Could you check a few things on this model? Use its own coordinates, in mm. A direction names the side the tool comes from. Coordinates: 2 decimals unless noted, no trailing zeros. Write each loop counter-clockwise with the first axis right and the second up, starting at its lowest first coordinate (ties: lowest second). Pieces come first, ordered by that corner, then holes.
Autodesk Inventor part; units mm, degrees
ref_plane "YZ Plane" through (0, 0, 0) normal (1, 0, 0) x (0, 1, 0)
ref_plane "XZ Plane" through (0, 0, 0) normal (0, 1, 0) x (-1, 0, 0)
ref_plane "XY Plane" through (0, 0, 0) normal (0, 0, 1) x (1, 0, 0)
sketch "Boceto1" plane through (0, 0, 0) normal (0, 0, 1) x (1, 0, 0)
  line L0 (-80, -30) -> (80, -30)
  line L1 (80, 30) -> (-80, 30)
  line L2 (-80, -30) -> (80, 30) construction
  line L3 (80, -30) -> (-80, 30) construction
  line L4 (0, -42) -> (0, 42) construction
  line L5 (-112, 0) -> (112, 0) construction
  arc A0 (-60, -10) -> (-60, 10) centre (-60, 0) ccw
  line L6 (-80, 10) -> (-60, 10)
  line L7 (-80, -10) -> (-60, -10)
  arc A1 (60, 10) -> (60, -10) centre (60, 0) ccw
  line L8 (80, 10) -> (60, 10)
  line L9 (80, -10) -> (60, -10)
  line L10 (-80, 30) -> (-80, 10)
  line L11 (-80, -10) -> (-80, -30)
  line L12 (80, -30) -> (80, -10)
  line L13 (80, 10) -> (80, 30)
  point P0 (0, 0)
  dimension "d2" = 160
  dimension "d3" = 60
  dimension "d4" = 20
  dimension "d6" = 20
  dimension "d7" = 20
extrude "Extrusión1" add sketch "Boceto1" along normal blind 20
sketch "Boceto2" plane through (0, 0, 20) normal (0, 0, 1) x (1, 0, 0)
  circle A0 centre (0, 0) radius 40
  dimension "d10" = 80
extrude "Extrusión2" add sketch "Boceto2" along normal blind 30 and the other way blind 20
sketch "Boceto3" plane through (0, 0, 50) normal (0, 0, 1) x (1, 0, 0)
  line L0 (-10, -20) -> (10, -20)
  line L1 (20, -10) -> (20, 10)
  line L2 (10, 20) -> (-10, 20)
  line L3 (-20, 10) -> (-20, -10)
  line L4 (-20, -20) -> (20, 20) construction
  line L5 (20, -20) -> (-20, 20) construction
  line L6 (-10, 20) -> (-20, 10)
  line L7 (10, 20) -> (20, 10)
  line L8 (20, -10) -> (10, -20)
  line L9 (-10, -20) -> (-20, -10)
  point P0 (0, 0)
  dimension "d15" = 40
  dimension "d16" = 40
  dimension "d17" = 10
  dimension "d18" = 10
  dimension "d19" = 10
  dimension "d20" = 10
  dimension "d21" = 10
  dimension "d22" = 10
  dimension "d23" = 10
  dimension "d24" = 10
extrude "Extrusión3" cut sketch "Boceto3" against normal through all
fillet "Empalme1" radius 10 4 edges at (80, 30, 10) (-80, 30, 10) (80, -30, 10) (-80, -30, 10)
equation "\"d18\" = d17"
equation "\"d19\" = d17"
equation "\"d20\" = d19"
equation "\"d21\" = d17"
equation "\"d22\" = d21"
equation "\"d23\" = d17"
equation "\"d24\" = d23"
properties part number "Lab2A01209499P10"
1. I want a section at A-A on y = 0. Please give me the cut outline in (x, z).
Verdict:
outline: (-50, 0) - (-20, 0) - (-20, 50) - (-40, 50) - (-40, 20) - (-50, 20) - close; (20, 0) - (50, 0) - (50, 20) - (40, 20) - (40, 50) - (20, 50) - close
2. I want a section at C-C on x = 0. Please give me the cut outline in (y, z), plus the area to 3 significant figures.
Verdict:
outline: (-40, 0) - (-20, 0) - (-20, 50) - (-40, 50) - close; (20, 0) - (40, 0) - (40, 50) - (20, 50) - close
area: 2,000 mm2
3. On a 3-axis mill with a long thin cutter (end or side, diameter ignored), from which of +Z, -Z, +X, -X, +Y, -Y can I reach the whole of each face in a straight line? I mean faces 5 (the face through (20, 0, 25)), 6 (the face through (48, -30, 10)), 7 (the face through (38.153, 12.015, 30.906)), 8 (the face through (-49, -30, 10)), 9 (the face through (70, 10, 10)). Say none if no direction works.
Verdict:
face 5: +Z, -Z
face 6: +Z, -Z, +X, -Y
face 7: +Z
face 8: +Z, -Z, -X, -Y
face 9: +Z, -Z, +X
4. If we mould it in two halves opening along Y, with no side actions, what happens to faces 1 (the face through (-15, -15, 25)), 2 (the face through (-76.99, 27.15, 10.14)), 3 (the face through (70, -10, 10)), 4 (the face through (-48, 0, 20))? For each: pulls with the +Y half, pulls with the -Y half, needs draft (parallel to the pull), parting line crosses it, or undercut.
Verdict:
face 1: undercut
face 2: pulls with the +Y half
face 3: undercut
face 4: needs draft
5. I want a section at B-B on z = 14.5. Please give me the cut outline in (x, y), plus the area to 3 significant figures.
Verdict:
outline: (-80, -20) arc R10 ccw to (-70, -30) - (-26.46, -30) arc R40 ccw to (26.46, -30) - (70, -30) arc R10 ccw to (80, -20) - (80, -10) - (60, -10) arc R10 cw to (60, 10) - (80, 10) - (80, 20) arc R10 ccw to (70, 30) - (26.46, 30) arc R40 ccw to (-26.46, 30) - (-70, 30) arc R10 ccw to (-80, 20) - (-80, 10) - (-60, 10) arc R10 cw to (-60, -10) - (-80, -10) - close; hole (-20, -10) - (-10, -20) - (10, -20) - (20, -10) - (20, 10) - (10, 20) - (-10, 20) - (-20, 10) - close
area: 7,730 mm2
6. Please list where these lines run through material, in increasing order: line 1 along Y through (x, z) = (45.5, 16.5); line 2 along Y through (x, z) = (65, 7.5); line 3 along X through (y, z) = (-15, 5).
Verdict:
line 1: y = -30 to 30
line 2: y = -30 to -10, 10 to 30
line 3: x = -80 to -15, 15 to 80
7. For pin 1 (10 mm diameter, centred on x = -61.5, z = 28, fed in from +Y); pin 2 (16 mm diameter, centred on x = -71, z = 14.5, fed in from +Y); pin 3 (2 mm diameter, centred on x = 55.5, y = 13.5, fed in from +Z); pin 4 (16 mm diameter, centred on x = 2.5, z = 23, fed in from +Y), each with a flat end and sliding along its axis, tell me the tip position at first contact or that it passes through.
Verdict:
pin 1: passes through
pin 2: stops at y = 30
pin 3: stops at z = 20
pin 4: stops at y = 40
8. I want a section at D-D on z = 36.5. Please give me the cut outline in (x, y), plus the area to 3 significant figures.
Verdict:
outline: circle Ø80 at (0, 0); hole (-20, -10) - (-10, -20) - (10, -20) - (20, -10) - (20, 10) - (10, 20) - (-10, 20) - (-20, 10) - close
area: 3,630 mm2
